```python
from build123d import *

# Parameters (mm, degrees)
SKETCH_1_R          = 13.25
EXTRUDE_1_DEPTH     = 3.5
SKETCH4_R           = 1.55
CUT_EXTRUDE5_DEPTH  = 5
SKETCH_2_R          = 2.1
CUT_EXTRUDE_1_DEPTH = 10
CUT_EXTRUDE_2_DEPTH = 171.144056611
FILLET_1_R          = 8
CUT_EXTRUDE_3_DEPTH = 3


with BuildPart() as part:
    # 草图1 → 凸台-拉伸1 (new, symmetric)
    with BuildSketch(Plane.XY):
        with BuildLine():
            Line((-19, 0), (19, 0))
            Line((19, 0), (19, 78.751923191))
            ThreePointArc((19, 78.751923191), (0, 120), (-19, 78.751923191))
            Line((-19, 78.751923191), (-19, 0))
        make_face()
        with BuildLine():
            ThreePointArc((-8, 9), (-5, 6), (-8, 3))
            Line((-8, 3), (-14, 3))
            ThreePointArc((-14, 3), (-17, 6), (-14, 9))
            Line((-14, 9), (-8, 9))
        make_face(mode=Mode.SUBTRACT)
        with BuildLine():
            ThreePointArc((8, 3), (5, 6), (8, 9))
            Line((8, 9), (14, 9))
            ThreePointArc((14, 9), (17, 6), (14, 3))
            Line((14, 3), (8, 3))
        make_face(mode=Mode.SUBTRACT)
        with BuildLine():
            ThreePointArc((-7.5, 65), (-5.303300859, 70.303300859), (0, 72.5))
            ThreePointArc((0, 72.5), (5.303300859, 70.303300859), (7.5, 65))
            Line((7.5, 65), (7.5, 20))
            ThreePointArc((7.5, 20), (0, 12.5), (-7.5, 20))
            Line((-7.5, 20), (-7.5, 65))
        make_face(mode=Mode.SUBTRACT)
        with Locations((0, 95)):
            Circle(SKETCH_1_R, mode=Mode.SUBTRACT)
    extrude(amount=EXTRUDE_1_DEPTH, both=True)

    # Sketch4 → Cut-Extrude5 (cut)
    with BuildSketch(Plane(origin=(0, 0, 0), x_dir=(-1, 0, 0), z_dir=(0, -1, 0))):
        with Locations(Location((11, 0, 0), (0, 0, 180))):
            Circle(SKETCH4_R)
        with Locations((-11, 0)):
            Circle(SKETCH4_R)
    extrude(amount=-CUT_EXTRUDE5_DEPTH, mode=Mode.SUBTRACT)

    # 草图2 → 切除-拉伸1 (cut)
    with BuildSketch(Plane.XY.offset(3.5)):
        with Locations((-18.5, 95)):
            Circle(SKETCH_2_R)
        with Locations((18.5, 95)):
            Circle(SKETCH_2_R)
    extrude(amount=-CUT_EXTRUDE_1_DEPTH, mode=Mode.SUBTRACT)

    # 草图4 → 切除-拉伸2 (cut, through all)
    with BuildSketch(Plane(origin=(0, 0, -114.5), x_dir=(-1, 0, 0), z_dir=(0, 0, -1))):
        with BuildLine():
            ThreePointArc((22.386292421, 106.128967232), (0.219572962, 119.999035736), (-22.187356595, 106.520469059))
            add(Edge.make_bspline(
                [(-22.187356595, 106.520469059), (0, 122.446847778), (22.386292421, 106.128967232)],
                knots=[0, 0, 0, 1, 1, 1], degree=2))
        make_face()
    extrude(amount=-CUT_EXTRUDE_2_DEPTH, mode=Mode.SUBTRACT)

    # 圆角1
    fillet_1_edges = [part.edges().sort_by_distance(p)[0] for p in [
        (-22.386292421, 106.128967232, 0),
        (22.187356595, 106.520469059, 0),
    ]]
    fillet(fillet_1_edges, radius=FILLET_1_R)

    # 草图5 → 切除-拉伸3 (cut)
    with BuildSketch(Plane.XY.offset(3.5)):
        Polygon((-22.238605802, 105.815360884), (0, 95), (-0.192853393, 99.54174681), (-22.228779927, 110.258538141), align=None)
        Polygon((-0.192853393, 99.54174681), (0, 95), (21.241716437, 107.661638988), (20.855269273, 112.087989547), align=None)
    extrude(amount=-CUT_EXTRUDE_3_DEPTH, mode=Mode.SUBTRACT)


solid = part.part
```
Verification items for the finished model (mm, model axes). A direction names the side the tool comes from. Coordinates: 2 decimals unless noted, no trailing zeros. Write each loop counter-clockwise with the first axis right and the second up, starting at its lowest first coordinate (ties: lowest second). Pieces come first, ordered by that corner, then holes. Notation, with made-up numbers: M 70,24.5 L 93,24.5 A23 cw 93,51.5 Z; hole C 22.25,41.25 d7. An arc over 180 degrees is marked long. Answer as a JSON object with one key per item and string values. Group by question number.
(1) Tool access check on faces 4 (the face through (19, 39, 0)), 5 (the face through (12.55, 1.48, -0.07)), 6 (the face through (-14.117, 106.313, 2.021)), 7 (the face through (0.16, 12.5, 0.05)). Record the directions out of +Z, -Z, +X, -X, +Y, -Y that give a thin tool (end or side, any length) a straight path to the whole face; none if there is none.
(2) Gauge pin test, flat ends, axial feed: pin 1 (3.5 mm diameter, centred on y = 51, z = 1, fed in from -X); pin 2 (3.5 mm diameter, centred on y = 39, z = 1.5, fed in from +X); pin 3 (2 mm diameter, centred on x = -3, z = -2, fed in from +Y); pin 4 (21 mm diameter, centred on x = 0, y = 95, fed in from +Z). Record the tip position at first contact, or that the pin passes through.
(3) Cross-section at B-B, the plane y = 6. Record the cut outline in (x, z).
(4) Release check for a two-part mould opening along X. For faces 1 (the face through (5, 71, -3.5)), 2 (the face through (-7.5, 42, 0)), 3 (the face through (-24.638, 90.762, 0.049)) record: +X half, -X half, draft (parallel to the pull), parting line (faces both ways), or undercut.
(5) Cross-section at D-D, the plane y = 76.5. Record the cut outline in (x, z).
(6) Cross-section at C-C, the plane x = 3. State how many separate pieces and enclosed holes the cut face has, and give its area (3 significant figures).
(7) Material ranges on line 1 (Y direction, x = 0.5, z = -0.5); line 2 (Z direction, x = 11, y = 1.05); line 3 (X direction, y = 36.5, z = 1.75), recorded low to high.
(8) Cross-section at A-A, the plane y = 44.5. Record the cut outline in (x, z), and give its area (3 significant figures).
Reply:
{
 "1": {"face 4": "+Z, -Z, +X, -Y", "face 5": "-Y", "face 6": "+Z", "face 7": "+Z, -Z"},
 "2": {"pin 1": "x = -19", "pin 2": "x = 19", "pin 3": "y = 114.31", "pin 4": "through"},
 "3": {"outline": "M -19,-3.5 L -17,-3.5 L -17,3.5 L -19,3.5 Z; M -5,-3.5 L 5,-3.5 L 5,3.5 L -5,3.5 Z; M 17,-3.5 L 19,-3.5 L 19,3.5 L 17,3.5 Z"},
 "4": {"face 1": "draft", "face 2": "undercut", "face 3": "-X half"},
 "5": {"outline": "M -19,-3.5 L 19,-3.5 L 19,3.5 L -19,3.5 Z"},
 "6": {"separate pieces": "3", "enclosed holes": "0", "area": "208 mm²"},
 "7": {"line 1": "0 to 12.52, 72.48 to 81.76, 108.24 to 114.39", "line 2": "-3.5 to -1.55, 1.55 to 3.5", "line 3": "-19 to -7.5, 7.5 to 19"},
 "8": {"outline": "M -19,-3.5 L -7.5,-3.5 L -7.5,3.5 L -19,3.5 Z; M 7.5,-3.5 L 19,-3.5 L 19,3.5 L 7.5,3.5 Z", "area": "161 mm²"}
}
